Work out the finished part from the listing and answer in its coordinate system (mm). A direction names the side the tool comes from. Coordinates: 2 decimals unless noted, no trailing zeros. Order: outer loops, then holes, each group sorted by start corner. A loop starts at its lowest first (then second) coordinate and runs counter-clockwise, first axis right, second up. Notation, with made-up numbers: (83, 58) - (131, 58) arc R9 cw to (131, 65) - close; hole circle Ø3 at (-19.5, 57). An arc over 180 degrees is marked (long way). Answer as a JSON object with one key per item and string values. Group by question number.
1) The mould has two halves that part along Z. Classify faces 3 (the face through (-15, 0, 1.588)), 4 (the face through (-0.014, -8.564, 15.146)), 5 (the face through (-1.016, -4, 13)): released by +Z, released by -Z, zero draft, split by the parting line, or undercut.
2) Each of these flat-tipped pins is pushed along its axis until it touches: P1, Ø11, axis at x = -19, y = -1, coming from the +Z side; P2, Ø7, axis at y = 2, z = 19, coming from the -X side; P3, Ø6, axis at y = -2.5, z = 10.5, coming from the +X side. Where does it stop, or does it pass through?
3) Section D-D (z = 12.25) is taken. Give the vertices of the cut face in (x, y).
4) Section A-A (y = -9.5) is taken. Give the vertices of the cut face in (x, z).
5) Section C-C (y = 4.25) is taken. Give the vertices of the cut face in (x, z), plus the area to 3 significant figures.
6) Find the intervals of material crossed by line 1 along Z through (x, y) = (16.5, 8.75); line 2 along X through (y, z) = (4, 11.25); line 3 along Y through (x, z) = (0.5, 2.5), in increasing order.
7) Section B-B (z = 25) is taken. Give the vertices of the cut face in (x, y), plus the area to 3 significant figures.
8) A tool of negligible diameter and unlimited length cuts with its end or side. For faces 1 (the face through (-25.4, 0, 1)), 2 (the face through (14, 0, 1.588)), from which of +Z, -Z, +X, -X, +Y, -Y can it reach the whole face along a straight path? Write none if from no direction.
from build123d import *

# Parameters (mm, degrees)
F0_W     = 50.8
F0_H     = 25.4
F1_DEPTH = 1.5875
F2_W     = 2.032
F2_H     = 25.4
F3_DEPTH = 25.4
F5_DEPTH = 25.4
F6_R     = 2.54
F7_R     = 2.54
F8_R     = 1.27
F9_DEPTH = 25.4


with BuildPart() as f1:
    # F0 (on Top) → F1 (new body)
    with BuildSketch(Plane.XY):
        Rectangle(F0_W, F0_H)
    extrude(amount=F1_DEPTH)

    # F2 (on face) → F3 (join)
    with BuildSketch(Plane.XY.offset(1.5875)):
        Rectangle(F2_W, F2_H)
    extrude(amount=F3_DEPTH)

    # F4 (on face) → F5 (cut)
    with BuildSketch(Plane(origin=(-1.016, 0, 0), x_dir=(0, -1, 0), z_dir=(-1, 0, 0))):
        Polygon((-12.7, 26.9875), (-12.7, 1.5875), (7.62, 26.9875), align=None)
    extrude(amount=-F5_DEPTH, mode=Mode.SUBTRACT)

    # F6
    f6_edges = [f1.edges().sort_by_distance(p)[0] for p in [
        (-1.016, 0, 1.5875),
        (1.016, 0, 1.5875),
    ]]
    fillet(f6_edges, radius=F6_R)

    # F7
    f7_edges = [f1.edges().sort_by_distance(p)[0] for p in [
        (0, -7.62, 26.9875),
        (0, -12.7, 26.9875),
    ]]
    fillet(f7_edges, radius=F7_R)

    # F8 (on face) → F9 (cut)
    with BuildSketch(Plane(origin=(-1.016, 0, 0), x_dir=(0, -1, 0), z_dir=(-1, 0, 0))):
        with Locations((9.5003935563, 24.4475)):
            Circle(F8_R)
        with Locations((9.5003935563, 19.3675)):
            Circle(F8_R)
        with Locations((9.5003935563, 14.2875)):
            Circle(F8_R)
        with Locations((9.5003935563, 9.2075)):
            Circle(F8_R)
    extrude(amount=-F9_DEPTH, mode=Mode.SUBTRACT)


solid = f1.part
Report:
{
 "1": {"face 3": "released by +Z", "face 4": "undercut", "face 5": "zero draft"},
 "2": {"P1": "stops at z = 1.59", "P2": "stops at x = -1.02", "P3": "stops at x = 1.02"},
 "3": {"outline": "(-1.02, -12.7) - (1.02, -12.7) - (1.02, 4.17) - (-1.02, 4.17) - close"},
 "4": {"outline": "(-25.4, 0) - (25.4, 0) - (25.4, 1.59) - (3.56, 1.59) arc R2.54 cw to (1.02, 4.13) - (1.02, 7.94) - (-1.02, 7.94) - (-1.02, 4.13) arc R2.54 cw to (-3.56, 1.59) - (-25.4, 1.59) - close; (-1.02, 10.48) - (1.02, 10.48) - (1.02, 13.02) - (-1.02, 13.02) - close; (-1.02, 15.56) - (1.02, 15.56) - (1.02, 18.1) - (-1.02, 18.1) - close; (-1.02, 20.64) - (1.02, 20.64) - (1.02, 23.18) - (-1.02, 23.18) - close; (-1.02, 25.72) - (1.02, 25.72) - (1.02, 26.99) - (-1.02, 26.99) - close"},
 "5": {"outline": "(-25.4, 0) - (25.4, 0) - (25.4, 1.59) - (3.56, 1.59) arc R2.54 cw to (1.02, 4.13) - (1.02, 12.15) - (-1.02, 12.15) - (-1.02, 4.13) arc R2.54 cw to (-3.56, 1.59) - (-25.4, 1.59) - close", "area": "105 mm²"},
 "6": {"line 1": "z = 0 to 1.59", "line 2": "x = -1.02 to 1.02", "line 3": "y = -12.7 to 11.97"},
 "7": {"outline": "(-1.02, -12.64) - (1.02, -12.64) - (1.02, -10.64) - (-1.02, -10.64) - close; (-1.02, -8.36) - (1.02, -8.36) - (1.02, -6.03) - (-1.02, -6.03) - close", "area": "8.78 mm²"},
 "8": {"face 1": "+Z, -Z, -X, +Y, -Y", "face 2": "+Z, +X, +Y, -Y"}
}
